```python
from build123d import *

# Parameters (mm, degrees)
MASS_DEPTH          = 6.35
SKETCH4_R           = 3.175
CUT_EXTRUDE1_DEPTH  = 122.586333782
SKETCH3_W           = 12.7
SKETCH3_H           = 12.7
CUT_EXTRUDE2_DEPTH  = 122.586333782
LPATTERN1_COUNT     = 7
LPATTERN1_PITCH     = 25.4
CAVITY1_START       = 59.53125
CAVITY1_OUTLINE_W   = 11.1125
CAVITY1_OUTLINE_H   = 6.35
CAVITY1_DEPTH       = 6.35
CAVITY1_START_2     = 88.9
CAVITY1_2_OUTLINE_W = 11.1125
CAVITY1_2_OUTLINE_H = 6.35
CAVITY1_2_DEPTH     = 6.35


# Read off the part's stored shape, not the designer's step: Cavity1
with BuildPart() as part:
    # Sketch1 → Mass (new body)
    with BuildSketch(Plane.XY):
        with BuildLine():
            Line((-95.25, -23.8125), (95.25, -23.8125))
            Line((95.25, -23.8125), (95.25, 23.8125))
            Line((95.25, 23.8125), (-95.25, 23.8125))
            ThreePointArc((-95.25, 23.8125), (-119.0625, 0), (-95.25, -23.8125))
        make_face()
    extrude(amount=MASS_DEPTH)

    # Sketch4 → Cut-Extrude1 (cut, through all)
    with BuildSketch(Plane(origin=(0, 0, 0), x_dir=(-1, 0, 0), z_dir=(0, 0, -1))):
        with Locations((95.25, 0)):
            Circle(SKETCH4_R)
    extrude(amount=-CUT_EXTRUDE1_DEPTH, mode=Mode.SUBTRACT)

    # Sketch3 → Cut-Extrude2 (cut, through all)
    with BuildSketch(Plane(origin=(0, 0, 0), x_dir=(-1, 0, 0), z_dir=(0, 0, -1))):
        with Locations((-88.9, 23.8125)):
            Rectangle(SKETCH3_W, SKETCH3_H)
        with Locations((-88.9, -23.8125)):
            Rectangle(SKETCH3_W, SKETCH3_H)
    cut_extrude2 = extrude(amount=-CUT_EXTRUDE2_DEPTH, mode=Mode.SUBTRACT)

    # LPattern1: Cut-Extrude2 ×7
    with Locations(*[(-i * LPATTERN1_PITCH, 0, 0) for i in range(1, LPATTERN1_COUNT)]):
        add(cut_extrude2, mode=Mode.SUBTRACT)

    # Cavity1 outline → Cavity1 (cut)
    with BuildSketch(Plane.YZ.offset(CAVITY1_START)):
        with Locations((-11.90625, 3.175)):
            Rectangle(CAVITY1_OUTLINE_W, CAVITY1_OUTLINE_H)
        with Locations((11.90625, 3.175)):
            Rectangle(CAVITY1_OUTLINE_W, CAVITY1_OUTLINE_H)
    extrude(amount=CAVITY1_DEPTH, mode=Mode.SUBTRACT)

    # Cavity1 2 outline → Cavity1 2 (cut)
    with BuildSketch(Plane.YZ.offset(CAVITY1_START_2)):
        with Locations((-11.90625, 3.175)):
            Rectangle(CAVITY1_2_OUTLINE_W, CAVITY1_2_OUTLINE_H)
        with Locations((11.90625, 3.175)):
            Rectangle(CAVITY1_2_OUTLINE_W, CAVITY1_2_OUTLINE_H)
    extrude(amount=CAVITY1_2_DEPTH, mode=Mode.SUBTRACT)


solid = part.part
```
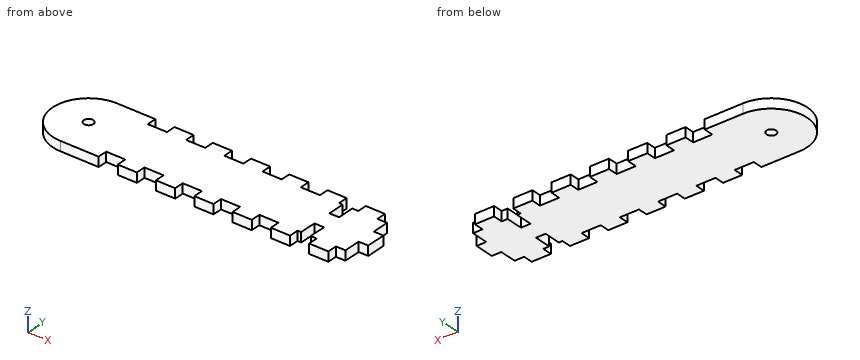
Build history of the part. All positions in model axes, mm. Round coordinates to 2 decimals unless told otherwise and drop trailing zeros. Write each loop counter-clockwise with the first axis right and the second up, starting at its lowest first coordinate (ties: lowest second). Pieces come first, ordered by that corner, then holes.
1) Drill centre lines: probe 1 along Y at (x, z) = (-95.25, 3.25) (1 decimal); probe 2 along Y at (x, z) = (60.5, 5.5); probe 3 along X at (y, z) = (9, 1.25). Where is each one in solid material? Low to high.
2) Band-saw the part on C-C, the plane y = -10. List the corners of the cut face in (x, z), and give its area (3 significant figures).
3) Pin check, flat tips, straight feed: pin 1 (1.9 mm diameter, centred on y = 14, z = 3, fed in from +X); pin 2 (1.9 mm diameter, centred on x = 12, z = 4, fed in from +Y); pin 3 (1.9 mm diameter, centred on y = 22, z = 2.5, fed in from -X). Stop position of each tip, or through.
4) Band-saw the part on B-B, the plane x = -12.5. List the corners of the cut face in (y, z), and give its area (3 significant figures).
Ans:
1. probe 1: y = -23.8 to -3.2, 3.2 to 23.8
1. probe 2: y = -6.35 to 6.35
1. probe 3: x = -117.3 to 59.53, 65.88 to 88.9
2. outline: (-116.86, 0) - (59.53, 0) - (59.53, 6.35) - (-116.86, 6.35) - close; (65.88, 0) - (88.9, 0) - (88.9, 6.35) - (65.88, 6.35) - close
2. area: 1,270 mm2
3. pin 1: stops at x = 88.9
3. pin 2: stops at y = 17.46
3. pin 3: stops at x = -106.38
4. outline: (-17.46, 0) - (17.46, 0) - (17.46, 6.35) - (-17.46, 6.35) - close
4. area: 222 mm2
